Could you check a few things on this model? Use its own coordinates, in mm. Give positions to 0.01 mm unless a question says otherwise; leave off trailing zeros. Order: outer loops, then holes, each group sorted by start corner. A loop starts at its lowest first (then second) coordinate and runs counter-clockwise, first axis right, second up. Notation, with made-up numbers: (7, 24) - (33, 24) arc R13 ccw to (33, 47) - close; hole circle Ø6 at (-39, 38.25). An arc over 180 degrees is marked (long way). One line per question, with ' | ' between items. Start each with the question number.
1. For P1, Ø2, axis at x = 0, y = 23, coming from the +Z side; P2, Ø14, axis at y = 91.5, z = 15.5, coming from the +X side; P3, Ø6, axis at x = -1, y = 76, coming from the -Z side; P4, Ø1, axis at x = 7, z = 22.5, coming from the -Y side, each with a flat end and sliding along its axis, tell me the tip position at first contact or that it passes through.
2. Imagine slicing it at C-C (z = 2.5). Please give me the cut outline in (x, y).
3. Imagine slicing it at A-A (z = 14). Please give me the cut outline in (x, y) (3 decimals), and give its area (3 significant figures).
4. Imagine slicing it at B-B (y = 89.5). Please give me the cut outline in (x, z) (3 decimals).
5. Imagine slicing it at D-D (y = 14). Please give me the cut outline in (x, z) (3 decimals), and give its area (3 significant figures).
6. I need wall thicknesses on probe 1 along X at (y, z) = (96, 9.5); probe 2 along Y at (x, z) = (6, 33). Which ranges of each line are inside material? Lowest first, please. Write a range as from..to.
Autodesk Inventor part; units mm, degrees
ref_plane "YZ Plane" through (0, 0, 0) normal (1, 0, 0) x (0, 1, 0)
ref_plane "XZ Plane" through (0, 0, 0) normal (0, 1, 0) x (-1, 0, 0)
ref_plane "XY Plane" through (0, 0, 0) normal (0, 0, 1) x (1, 0, 0)
sketch "Sketch1" plane through (0, 0, 0) normal (0, 0, 1) x (1, 0, 0)
  line L0 (0, 0) -> (6.35, 0)
  line L1 (6.35, 0) -> (6.35, 101.6)
  line L2 (6.35, 101.6) -> (0, 101.6)
  line L3 (0, 101.6) -> (0, 0)
  dimension "d0" = 6.35
  dimension "d1" = 101.6
extrude "Extrusion1" add sketch "Sketch1" along normal blind 6.35
sketch "Sketch2" plane through (6.35, 0, 0) normal (1, 0, 0) x (0, 0, -1)
  line L0 (-19.05, 0) -> (-25.4, 0)
  line L1 (-25.4, 0) -> (-6.35, 19.05)
  line L2 (-6.35, 0) -> (-6.35, 101.6)
  line L3 (-25.4, 0) -> (1.5408, 0) construction
  line L4 (-6.35, 19.05) -> (-6.35, 12.7)
  line L5 (-6.35, 12.7) -> (-19.05, 0)
  point P0 (0, 0)
  dimension "d5" = 19.05
  dimension "d6" = 45
  dimension "d7" = 6.35
extrude "Extrusion2" add sketch "Sketch2" against normal blind 6.35
sketch "Sketch3" plane through (6.35, 0, 0) normal (1, 0, 0) x (0, 0, -1)
  line L0 (12.7, 0) -> (19.05, 0)
  line L1 (19.05, 0) -> (0, 19.05)
  line L2 (0, 101.6) -> (0, 0)
  line L3 (0, 19.05) -> (0, 12.7)
  line L4 (0, 12.7) -> (12.7, 0)
  dimension "d10" = 19.05
  dimension "d11" = 45
  dimension "d12" = 6.35
extrude "Extrusion3" add sketch "Sketch3" against normal blind 6.35
sketch "Sketch4" plane through (0, 0, 6.35) normal (0, 0, 1) x (1, 0, 0)
  line L0 (6.35, 19.05) -> (25.4, 0)
  line L1 (6.35, 19.05) -> (33.2908, 19.05) construction
  line L2 (25.4, 0) -> (19.05, 0)
  line L3 (0, 0) -> (6.35, 0)
  line L4 (19.05, 0) -> (6.35, 12.7)
  line L5 (6.35, 12.7) -> (6.35, 19.05)
  line L6 (6.35, 0) -> (6.35, 12.7)
  dimension "d15" = 45
  dimension "d16" = 6.35
extrude "Extrusion4" add sketch "Sketch4" against normal blind 6.35
sketch "Sketch5" plane through (0, 0, 0) normal (0, 0, -1) x (-1, 0, 0)
  line L0 (0, 19.05) -> (19.05, 0)
  line L1 (0, 19.05) -> (26.9408, 19.05) construction
  line L2 (19.05, 0) -> (12.7, 0)
  line L3 (0, 19.05) -> (0, 0)
  line L4 (12.7, 0) -> (0, 12.7)
  line L5 (0, 12.7) -> (0, 19.05)
  dimension "d19" = 45
  dimension "d20" = 6.35
extrude "Extrusion5" add sketch "Sketch5" against normal blind 6.35
sketch "Sketch6" plane through (6.35, 101.6, 6.35) normal (1, 0, 0) x (0, 0, -1)
  line L0 (0, 0) -> (-50.8, 0)
  line L1 (-50.8, 0) -> (-50.8, -6.35)
  line L2 (-50.8, -6.35) -> (0, -6.35)
  line L3 (0, -6.35) -> (0, 0)
  line L4 (6.35, 0) -> (25.4, 0)
  line L5 (25.4, 0) -> (25.4, -6.35)
  line L6 (25.4, -6.35) -> (6.35, -6.35)
  line L7 (6.35, -6.35) -> (6.35, 0)
  point P0 (6.35, -101.6)
  dimension "d23" = 50.8
  dimension "d24" = 6.35
  dimension "d25" = 19.05
extrude "Extrusion6" add sketch "Sketch6" against normal blind 6.35
sketch "Sketch7" plane through (6.35, 19.05, 6.35) normal (1, 0, 0) x (0, 0, -1)
  line L0 (-8.89, 76.2) -> (-12.7, 76.2)
  line L1 (-50.8, 76.2) -> (0, 76.2)
  line L2 (-12.7, 76.2) -> (0, 63.5)
  line L3 (0, 0) -> (0, 76.2)
  line L4 (0, 63.5) -> (0, 67.31)
  line L5 (0, 67.31) -> (-8.89, 76.2)
  point P0 (6.35, -19.05)
  dimension "d28" = 12.7
  dimension "d29" = 45
  dimension "d30" = 3.81
extrude "Extrusion7" add sketch "Sketch7" against normal blind 5.715 contours L5 L3 L2 L0
extrude "Extrusion8" cut sketch "Sketch7" against normal blind 0.635 contours L5 L3 L2 L0
sketch "Sketch9" plane through (0, 0, 6.35) normal (0, 0, 1) x (1, 0, 0)
  point P0 (0, 0)
extrude "Extrusion9" cut sketch "Sketch4" against normal blind 0.635
sketch "Sketch10" plane through (0, 0, 0) normal (0, 0, -1) x (-1, 0, 0)
  line L0 (-25.4, 0) -> (-19.05, 0)
  line L1 (-25.4, 0) -> (-19.05, 0)
  line L2 (-19.05, 0) -> (-6.35, 12.7)
  line L3 (-19.05, 0) -> (-6.35, 12.7)
  line L4 (-6.35, 12.7) -> (-6.35, 19.05)
  line L5 (-6.35, 0) -> (-6.35, 19.05)
  line L6 (-6.35, 19.05) -> (-25.4, 0)
  line L7 (-6.35, 19.05) -> (-25.4, 0)
  point P0 (0, 0)
extrude "Extrusion10" cut sketch "Sketch10" against normal blind 0.635
sketch "Sketch11" plane through (6.35, 0, 6.35) normal (1, 0, 0) x (0, 0, -1)
  line L0 (6.35, 19.05) -> (6.35, 12.7)
  line L1 (6.35, 0) -> (6.35, 12.7)
  line L2 (6.35, 12.7) -> (19.05, 0)
  line L3 (6.35, 12.7) -> (19.05, 0)
  line L4 (19.05, 0) -> (25.4, 0)
  line L5 (19.05, 0) -> (25.4, 0)
  line L6 (25.4, 0) -> (6.35, 19.05)
  line L7 (25.4, 0) -> (6.35, 19.05)
extrude "Extrusion11" cut sketch "Sketch11" against normal blind 0.635
sketch "Sketch12" plane through (0, 0, -19.05) normal (-1, 0, 0) x (0, 0, 1)
  line L0 (0, 0) -> (6.35, 0)
  line L1 (0, 0) -> (6.35, 0)
  line L2 (6.35, 0) -> (19.05, 12.7)
  line L3 (6.35, 0) -> (19.05, 12.7)
  line L4 (19.05, 12.7) -> (19.05, 19.05)
  line L5 (19.05, 95.25) -> (19.05, 19.05)
  line L6 (19.05, 19.05) -> (0, 0)
  line L7 (19.05, 19.05) -> (0, 0)
  point P0 (19.05, 0)
extrude "Extrusion12" cut sketch "Sketch12" against normal blind 0.635
sketch "Sketch13" plane through (0, 0, 0) normal (0, 0, -1) x (-1, 0, 0)
  line L0 (0, 19.05) -> (0, 12.7)
  line L1 (0, 12.7) -> (12.7, 0)
  line L2 (0, 12.7) -> (12.7, 0)
  line L3 (12.7, 0) -> (19.05, 0)
  line L4 (19.05, 0) -> (0, 19.05)
  line L5 (19.05, 0) -> (0, 19.05)
  point P0 (0, 0)
extrude "Extrusion13" cut sketch "Sketch13" against normal blind 0.635
sketch "Sketch14" plane through (0, 0, 6.35) normal (0, 0, 1) x (1, 0, 0)
  line L0 (-19.05, 0) -> (-12.7, 0)
  line L1 (-19.05, 0) -> (-12.7, 0)
  line L2 (-12.7, 0) -> (0, 12.7)
  line L3 (-12.7, 0) -> (0, 12.7)
  line L4 (0, 12.7) -> (0, 19.05)
  line L5 (0, 12.7) -> (0, 19.05)
  line L6 (0, 19.05) -> (-19.05, 0)
  line L7 (0, 19.05) -> (-19.05, 0)
  point P0 (0, 0)
extrude "Extrusion14" cut sketch "Sketch14" against normal blind 0.635
sketch "Sketch15" plane through (0, 0, 0) normal (-1, 0, 0) x (0, 0, 1)
  line L0 (6.35, 19.05) -> (25.4, 0)
  line L1 (6.35, 19.05) -> (25.4, 0)
  line L2 (25.4, 0) -> (19.05, 0)
  line L3 (25.4, 0) -> (19.05, 0)
  line L4 (19.05, 0) -> (6.35, 12.7)
  line L5 (6.35, 12.7) -> (6.35, 19.05)
  point P0 (0, 0)
extrude "Extrusion15" cut sketch "Sketch15" against normal blind 0.635
sketch "Sketch16" plane through (6.35, 0, 6.35) normal (1, 0, 0) x (0, 0, -1)
  line L0 (-19.05, 0) -> (-12.7, 0)
  line L1 (-19.05, 0) -> (-12.7, 0)
  line L2 (-12.7, 0) -> (0, 12.7)
  line L3 (0, 19.05) -> (-19.05, 0)
  line L4 (0, 12.7) -> (0, 19.05)
  line L5 (0, 95.25) -> (0, 0)
  line L6 (0, 19.05) -> (-19.05, 0)
  point P0 (6.35, 0)
extrude "Extrusion16" cut sketch "Sketch16" against normal blind 0.635
sketch "Sketch17" plane through (6.35, 0, 6.35) normal (1, 0, 0) x (0, 0, -1)
  line L0 (15.24, 95.25) -> (19.05, 95.25)
  line L1 (25.4, 95.25) -> (6.35, 95.25)
  line L2 (19.05, 95.25) -> (6.35, 82.55)
  line L3 (6.35, 0) -> (6.35, 95.25)
  line L4 (6.35, 82.55) -> (6.35, 86.36)
  line L5 (6.35, 86.36) -> (15.24, 95.25)
  line L6 (6.35, 86.36) -> (18.9224, 86.36) construction
  dimension "d51" = 12.7
  dimension "d52" = 45
  dimension "d53" = 45
extrude "Extrusion17" add sketch "Sketch17" against normal blind 5.715 contours L0 L2 L3 L5
sketch "Sketch18" plane through (6.35, 0, 6.35) normal (1, 0, 0) x (0, 0, -1)
  line L0 (6.35, 86.36) -> (6.35, 82.55)
  line L1 (6.35, 95.25) -> (6.35, 0)
  line L2 (6.35, 82.55) -> (19.05, 95.25)
  line L3 (19.05, 95.25) -> (6.35, 82.55)
  line L4 (19.05, 95.25) -> (15.24, 95.25)
  line L5 (25.4, 95.25) -> (6.35, 95.25)
  line L6 (15.24, 95.25) -> (6.35, 86.36)
  line L7 (15.24, 95.25) -> (6.35, 86.36)
extrude "Extrusion18" cut sketch "Sketch18" against normal blind 0.635 contours L6 L4 L2 L0
sketch "Sketch19" plane through (6.35, 0, 6.35) normal (1, 0, 0) x (0, 0, -1)
  line L0 (25.4, 101.6) -> (-50.8, 101.6)
  line L1 (-50.8, 95.25) -> (0, 95.25)
  line L2 (-44.45, 101.6) -> (-41.91, 101.6)
  line L3 (-41.91, 101.6) -> (-41.91, 95.25)
  line L4 (-41.91, 95.25) -> (-44.45, 95.25)
  line L5 (-44.45, 95.25) -> (-44.45, 101.6)
  point P0 (6.35, 0)
  dimension "d58" = 6.35
  dimension "d59" = 2.54
extrude "Extrusion19" cut sketch "Sketch19" against normal blind 0.635
sketch "Sketch20" plane through (0, 101.6, -19.05) normal (0, 1, 0) x (1, 0, 0)
  line L0 (0, -25.4) -> (0, -76.2)
  line L1 (5.715, -67.31) -> (0, -67.31)
  line L2 (0, -67.31) -> (0, -69.85)
  line L3 (0, -69.85) -> (5.715, -69.85)
  line L4 (5.715, -69.85) -> (5.715, -67.31)
  point P0 (0, -19.05)
extrude "Extrusion20" cut sketch "Sketch20" against normal blind 0.635
sketch "Sketch21" plane through (0, 0, 0) normal (-1, 0, 0) x (0, 0, 1)
  line L0 (50.8, 100.965) -> (48.26, 100.965)
  line L1 (48.26, 100.965) -> (48.26, 95.25)
  line L2 (48.26, 95.25) -> (50.8, 95.25)
  line L3 (50.8, 95.25) -> (50.8, 100.965)
  point P0 (0, 0)
extrude "Extrusion21" cut sketch "Sketch21" against normal blind 0.635
sketch "Sketch22" plane through (0, 95.25, 6.35) normal (0, -1, 0) x (1, 0, 0)
  line L0 (0.635, 41.91) -> (5.715, 41.91)
  line L1 (5.715, 41.91) -> (5.715, 44.45)
  line L2 (5.715, 44.45) -> (0.635, 44.45)
  line L3 (0.635, 44.45) -> (0.635, 41.91)
  point P0 (0, -6.35)
extrude "Extrusion22" cut sketch "Sketch22" against normal blind 0.635
fillet "Fillet1" radius 0.635 8 edges at (3.175, 100.965, 48.26) (5.715, 98.425, 48.26) (3.175, 100.965, 50.8) (5.715, 98.425, 50.8) (0.635, 98.425, 48.26) (3.175, 95.885, 48.26) (0.635, 98.425, 50.8) (3.175, 95.885, 50.8)
fillet "Fillet2" radius 0.635 12 edges at (0.4492, 95.6992, 50.6142) (0.4492, 95.6992, 48.4458) (0.635, 95.885, 49.53) (0.4492, 101.1508, 50.6142) (0.4492, 101.1508, 48.4458) (0.635, 100.965, 49.53) (5.9008, 95.6992, 48.4458) (5.9008, 95.6992, 50.6142) (5.715, 95.885, 49.53) (5.9008, 101.1508, 50.6142) (5.9008, 101.1508, 48.4458) (5.715, 100.965, 49.53)
properties part number "Gallows 1" material "Wood (Birch)"
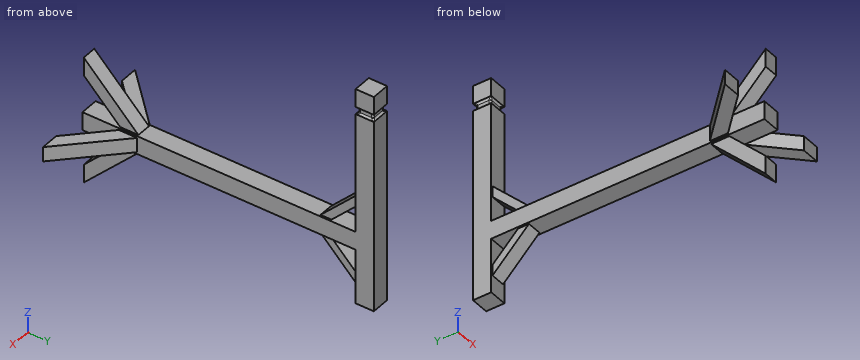
Results found:
1) P1: stops at z = 6.35 | P2: stops at x = 6.35 | P3: stops at z = 0 | P4: passes through
2) outline: (-19.05, 0) - (-12.7, 0) - (0, 12.7) - (0, 0) - (6.35, 0) - (6.35, 12.7) - (19.05, 0) - (25.4, 0) - (6.35, 19.05) - (6.35, 101.6) - (0, 101.6) - (0, 19.05) - close
3) outline: (0, 95.25) - (6.35, 95.25) - (6.35, 101.6) - (0, 101.6) - close; (0.635, 5.05) - (5.715, 5.05) - (5.715, 11.4) - (0.635, 11.4) - close; (0.635, 90.2) - (5.715, 90.2) - (5.715, 94.01) - (0.635, 94.01) - close | area: 91.9 mm2
4) outline: (0, 0) - (6.35, 0) - (6.35, 6.35) - (0, 6.35) - close; (0.635, -6.95) - (5.715, -6.95) - (5.715, -3.14) - (0.635, -3.14) - close; (0.635, 9.49) - (5.715, 9.49) - (5.715, 13.3) - (0.635, 13.3) - close
5) outline: (-5.05, 0.635) - (0, 0.635) - (0, 0) - (0.635, 0) - (0.635, -5.05) - (5.715, -5.05) - (5.715, 0) - (6.35, 0) - (6.35, 0.635) - (11.4, 0.635) - (11.4, 5.715) - (6.35, 5.715) - (6.35, 6.35) - (5.715, 6.35) - (5.715, 11.4) - (0.635, 11.4) - (0.635, 6.35) - (0, 6.35) - (0, 5.715) - (-5.05, 5.715) - close | area: 143 mm2
6) probe 1: x = 0..6.35 | probe 2: y = 95.25..101.6
